```python
from build123d import *

# Parameters (mm, degrees)
SKETCH_1_R               = 5
EXTRUDE_1_DEPTH          = 100
SKETCH_2_R               = 12.5
EXTRUDE_2_DEPTH          = 1
PATTERN_LINEAR_1_COUNT   = 3
PATTERN_LINEAR_1_PITCH   = 35
PATTERN_LINEAR_2_COUNT   = 3
PATTERN_LINEAR_2_PITCH   = 35
SKETCH_3_R               = 1.5
CUT_EXTRUDE_1_DEPTH      = 499.5
PATTERN_CIRCULAR_1_COUNT = 4


with BuildPart() as part:
    # 草图1 → 凸台-拉伸1 (new, symmetric)
    with BuildSketch(Plane(origin=(0, 0, 0), x_dir=(0, 0, -1), z_dir=(1, 0, 0))):
        Circle(SKETCH_1_R)
    extrude(amount=EXTRUDE_1_DEPTH, both=True)

    # 草图2 → 凸台-拉伸2 (add, symmetric)
    with BuildSketch(Plane(origin=(0, 0, 0), x_dir=(0, 0, -1), z_dir=(1, 0, 0))):
        Circle(SKETCH_2_R)
    extrude_2 = extrude(amount=EXTRUDE_2_DEPTH, both=True)

    # 阵列(线性)1: 凸台-拉伸2 ×3
    with Locations(*[(-i * PATTERN_LINEAR_1_PITCH, 0, 0) for i in range(1, PATTERN_LINEAR_1_COUNT)]):
        add(extrude_2)

    # 阵列(线性)2: 凸台-拉伸2 ×3
    with Locations(*[(i * PATTERN_LINEAR_2_PITCH, 0, 0) for i in range(1, PATTERN_LINEAR_2_COUNT)]):
        add(extrude_2)

    # 草图3 → 切除-拉伸1 (cut, symmetric)
    with BuildSketch(Plane(origin=(1, 0, 0), x_dir=(0, 0, -1), z_dir=(1, 0, 0))):
        with Locations((2.5, 10)):
            Circle(SKETCH_3_R)
        with Locations((-2.5, 10)):
            Circle(SKETCH_3_R)
    cut_extrude_1 = extrude(amount=CUT_EXTRUDE_1_DEPTH, both=True, mode=Mode.SUBTRACT)

    # 阵列(圆周)1: 切除-拉伸1 ×4 about axis
    pattern_circular_1_axis = Axis((0, 0, 0), (1, 0, 0))
    for i in range(1, PATTERN_CIRCULAR_1_COUNT):
        add(cut_extrude_1.rotate(pattern_circular_1_axis, i * 360 / PATTERN_CIRCULAR_1_COUNT), mode=Mode.SUBTRACT)


solid = part.part
```
Verification items for the finished model (mm, model axes). A direction names the side the tool comes from. Coordinates: 2 decimals unless noted, no trailing zeros. Loops run counter-clockwise (first coordinate to the right, second up) from the corner with the lowest first, then second, coordinate; pieces in that order, holes last. Notation, with made-up numbers: (-1, 28.25) -> (54, 28.25) arc R33 cw to (54, 67.25) -> close; hole circle Ø2 at (0.25, -37). An arc over 180 degrees is marked (long way). Answer in a Markdown table with one row per item. Add a question column.
1. Draft check along X on faces 4 (the face through (71, -5.4, 0.2)), 5 (the face through (-1, -5.4, 0.2)), 6 (the face through (-71, -5.4, 0.2)). Enter one of: +X half, -X half, draft (parallel to the pull), parting line (faces both ways), or undercut.
2. Material ranges on probe 1 along X at (y, z) = (-9.5, -5); probe 2 along Y at (x, z) = (0.55, 2.5), recorded low to high. Write a range as [from, to].
3. Depth check by flat-ended pin: P1, Ø5, axis at y = -10, z = -2.5, coming from the -X side; P2, Ø2.5, axis at y = 10, z = 2.5, coming from the -X side; P3, Ø3.5, axis at y = -10, z = 2.5, coming from the +X side; P4, Ø1.5, axis at x = -4.5, y = 4.5, coming from the +Z side. Enter the tip coordinate at first touch or a pass-through.
4. Access from +Z, -Z, +X, -X, +Y, -Y to the whole of each face (thin tool, end or side, straight path). Record for faces 1 (the face through (85.7, -4.88, 1.08)), 2 (the face through (-36, -5.4, 0.2)), 3 (the face through (0.014, 3.755, -11.923)).
5. Section check A-A, the plane x = 19. Enter the section's corners in (y, z).
Derived:
| question | item | result |
|---|---|---|
| 1 | face 4 | +X half |
| 1 | face 5 | undercut |
| 1 | face 6 | -X half |
| 2 | probe 1 | x = [-71, -69], [-36, -34], [-1, 1], [34, 36], [69, 71] |
| 2 | probe 2 | y = [-12.25, -11.5], [-8.5, 8.5], [11.5, 12.25] |
| 3 | P1 | stops at x = -71 |
| 3 | P2 | passes through |
| 3 | P3 | stops at x = 71 |
| 3 | P4 | stops at z = 3.31 |
| 4 | face 1 | +X |
| 4 | face 2 | none |
| 4 | face 3 | +X, -X |
| 5 | outline | circle Ø10 at (0, 0) |
